from build123d import *

# Parameters (mm, degrees)
SKETCH1_R                = 7.5
BOSS_EXTRUDE2_DEPTH      = 10
SKETCH3_W                = 11.5
SKETCH3_H                = 162
BOSS_EXTRUDE3_DEPTH      = 0.001
BOSS_EXTRUDE3_DEPTH_BACK = 10
SKETCH4_W                = 10.001
SKETCH4_H                = 6.029708674
BOSS_EXTRUDE4_DEPTH      = 40
BOSS_EXTRUDE4_DEPTH_BACK = 48
FILLET1_R                = 10
FILLET2_R                = 10
FILLET3_R                = 5
FILLET4_R                = 5
FILLET5_R                = 5
FILLET6_R                = 5


with BuildPart() as part:
    # Sketch1 → Boss-Extrude2 (new body)
    with BuildSketch(Plane.XY):
        Circle(SKETCH1_R)
    extrude(amount=BOSS_EXTRUDE2_DEPTH)

    # Sketch3 → Boss-Extrude3 (add, two sides)
    with BuildSketch(Plane.XY.offset(10)) as boss_extrude3_sk:
        with Locations((-0.261803669, -85.484218622)):
            Rectangle(SKETCH3_W, SKETCH3_H)
    extrude(amount=BOSS_EXTRUDE3_DEPTH)
    extrude(boss_extrude3_sk.sketch, amount=-BOSS_EXTRUDE3_DEPTH_BACK)

    # Sketch4 → Boss-Extrude4 (add, two sides)
    with BuildSketch(Plane(origin=(5.488196331, 0, 0), x_dir=(0, 0, -1), z_dir=(1, 0, 0))) as boss_extrude4_sk:
        with Locations((-5.0005, -163.469364285)):
            Rectangle(SKETCH4_W, SKETCH4_H)
    extrude(amount=BOSS_EXTRUDE4_DEPTH)
    extrude(boss_extrude4_sk.sketch, amount=-BOSS_EXTRUDE4_DEPTH_BACK)

    # Fillet1
    fillet1_edges = [part.edges().sort_by_distance(p)[0] for p in [
        (5.488196331, -5.111721924, 5),
    ]]
    fillet(fillet1_edges, radius=FILLET1_R)

    # Fillet2
    fillet2_edges = [part.edges().sort_by_distance(p)[0] for p in [
        (-6.011803669, -4.484218622, 5),
    ]]
    fillet(fillet2_edges, radius=FILLET2_R)

    # Fillet3
    fillet3_edges = [part.edges().sort_by_distance(p)[0] for p in [
        (5.488196331, -160.454509948, 5.0005),
    ]]
    fillet(fillet3_edges, radius=FILLET3_R)

    # Fillet4
    fillet4_edges = [part.edges().sort_by_distance(p)[0] for p in [
        (-6.011803669, -160.454509948, 5.0005),
    ]]
    fillet(fillet4_edges, radius=FILLET4_R)

    # Fillet5
    fillet5_edges = [part.edges().sort_by_distance(p)[0] for p in [
        (-42.511803669, -160.454509948, 5.0005),
    ]]
    fillet(fillet5_edges, radius=FILLET5_R)

    # Fillet6
    fillet6_edges = [part.edges().sort_by_distance(p)[0] for p in [
        (45.488196331, -160.454509948, 5.0005),
    ]]
    fillet(fillet6_edges, radius=FILLET6_R)


solid = part.part
Verification items for the finished model (mm, model axes). A direction names the side the tool comes from. Coordinates: 2 decimals unless noted, no trailing zeros. Order: outer loops, then holes, each group sorted by start corner. A loop starts at its lowest first (then second) coordinate and runs counter-clockwise, first axis right, second up.
1. Release check for a two-part mould opening along Y. For faces 1 (the face through (5.788, -5.716, 4.93)), 2 (the face through (-2, -98, 10.001)), 3 (the face through (25, -160.455, 5)), 4 (the face through (0.47, 7.485, 4.93)) record: +Y half, -Y half, draft (parallel to the pull), parting line (faces both ways), or undercut.
Results found:
face 1: undercut
face 2: draft
face 3: +Y half
face 4: undercut
2. Scan lines: line 1 (X direction, y = -127, z = 0.75); line 2 (Y direction, x = 33, z = 2.25); line 3 (X direction, y = -2, z = 3). Record each from-to range of solid material in increasing order.
Results found:
line 1: x = -6.01 to 5.49
line 2: y = -166.48 to -160.45
line 3: x = -7.23 to 7.23
3. Set-up check for faces 5 (the face through (-24, -160.455, 5)), 6 (the face through (-7.438, -158.951, 4.93)), 7 (the face through (5.488, -81, 5)): record each of +Z, -Z, +X, -X, +Y, -Y from which the full face is reachable in a straight line by a thin tool's end or side.
Results found:
face 5: +Z, -Z, -X, +Y
face 6: +Z, -Z, -X
face 7: +Z, -Z, +X
4. Sectioned sample at B-B, the plane y = -58. Record the cut outline in (x, z).
Results found:
outline: (-6.01, 0) - (5.49, 0) - (5.49, 10) - (-6.01, 10) - close
5. Go/stop test with a flat-tipped pin: pin 1 Ø1 at (x, z) = (15, 4.5) entering from +Y. Record where the tip stops, or that it passes through.
Results found:
pin 1: stops at y = -160.45
6. Sectioned sample at A-A, the plane z = 6.5. Record the cut outline in (x, y), and give its area (3 significant figures).
Results found:
outline: (-42.51, -166.48) - (45.49, -166.48) - (45.49, -165.45) arc R5 ccw to (40.49, -160.45) - (10.49, -160.45) arc R5 cw to (5.49, -155.45) - (5.49, -8.15) arc R10 cw to (6.64, -3.49) arc R7.5 ccw (long way) to (-6.86, -3.03) arc R10 cw to (-6.01, -7.06) - (-6.01, -155.45) arc R5 cw to (-11.01, -160.45) - (-37.51, -160.45) arc R5 ccw to (-42.51, -165.45) - close
area: 2,480 mm2
7. Sectioned sample at C-C, the plane x = 38. Record the cut outline in (y, z), and give its area (3 significant figures).
Results found:
outline: (-166.48, 0) - (-160.45, 0) - (-160.45, 10) - (-166.48, 10) - close
area: 60.3 mm2
